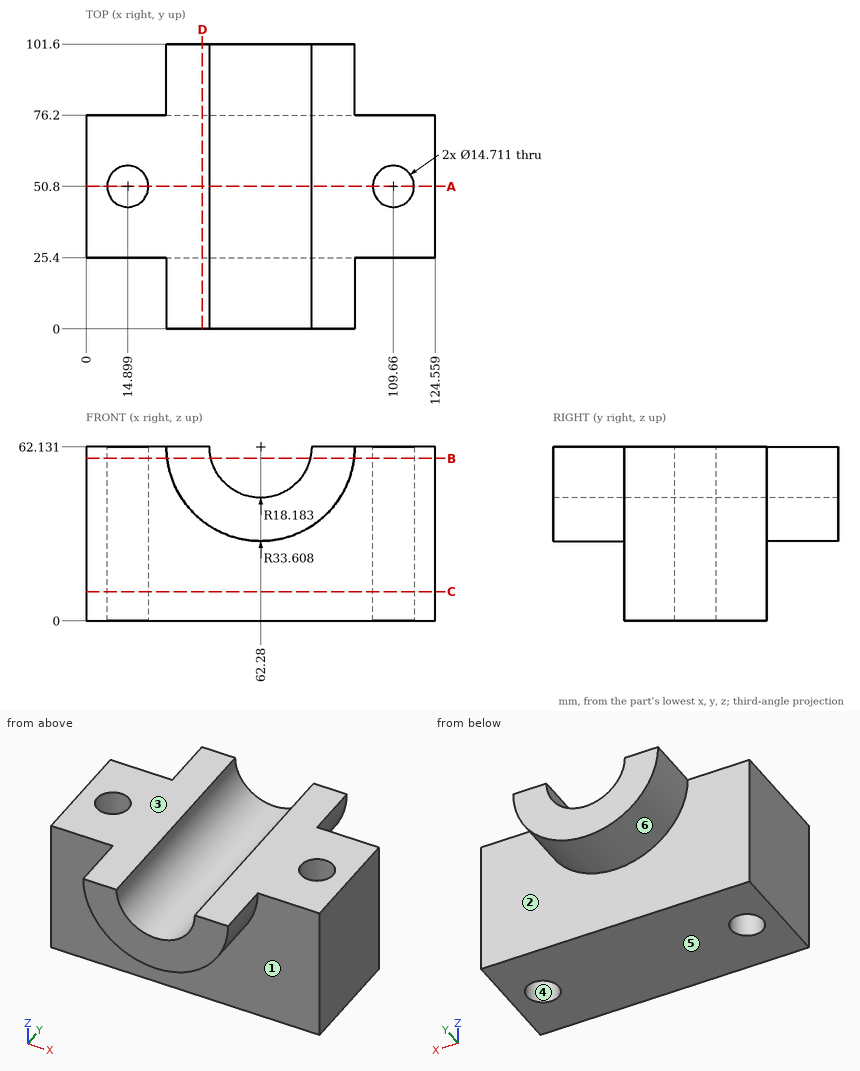
For this review, use the dimensioned drawing (mm, ordinates from the lowest corner) and the shaded views. A direction names the side the tool comes from. Round coordinates to 2 decimals unless told otherwise and drop trailing zeros. Order: outer loops, then holes, each group sorted by start corner. A loop starts at its lowest first (then second) coordinate and runs counter-clockwise, first axis right, second up. Notation, with made-up numbers: (85.25, -26.5) -> (97.25, -26.5) arc R24 ccw to (97.25, -4.5) -> close; hole circle Ø11 at (85, 3). An arc over 180 degrees is marked (long way). Use CSV: the item, a comma, the result in double quotes. Start each with the question number.
(1) Mouldability with a two-part tool opening along X and no side actions: class the marked faces 4, 5 and 6 as pulls with the +X half, pulls with the -X half, needs draft (parallel to the pull), parting line crosses it, or undercut.
(2) Consider section A-A on y = 50.8. Write out the cut boundary in (x, z) (1 decimal).
(3) Consider section D-D on x = 41.5. Write out the cut boundary in (y, z), and give its area (3 significant figures).
(4) Consider section B-B on z = 58. Write out the cut boundary in (x, y) (1 decimal).
(5) Tool access review of the marked faces 1, 2 and 3: name each direction out of +Z, -Z, +X, -X, +Y, -Y from which nothing blocks a thin tool from reaching the whole face with its end or side.
(6) Insertion check: pin 1 (2 mm diameter, centred on x = 71, y = 19, fed in from +Z) (1 decimal); pin 2 (13 mm diameter, centred on x = 109.66, y = 50.8, fed in from +Z); pin 3 (10 mm diameter, centred on y = 19, z = 37.5, fed in from -X); pin 4 (3 mm diameter, centred on x = 17, z = 16, fed in from -Y). Each pin has a flat end and moves straight along its axis. Give the tip position at first contact, or say it passes through.
(7) Wall thickness on probe 1 along X at (y, z) = (50.5, 30.5); probe 2 along X at (y, z) = (57.5, 31) (1 decimal); probe 3 along Y at (x, z) = (16, 40): over which ranges is each line inside the solid? List them lowest first. Write a range as from..to.
(8) Consider section C-C on z = 10.5. Write out the cut boundary in (x, y) (1 decimal).
Responses:
1,face 4,"undercut"
1,face 5,"needs draft"
1,face 6,"parting line crosses it"
2,outline,"(0, 0) -> (7.5, 0) -> (7.5, 62.1) -> (0, 62.1) -> close; (22.3, 0) -> (102.3, 0) -> (102.3, 62.1) -> (80.5, 62.1) arc R18.2 cw to (44.1, 62.1) -> (22.3, 62.1) -> close; (117, 0) -> (124.6, 0) -> (124.6, 62.1) -> (117, 62.1) -> close"
3,outline,"(0, 35.72) -> (25.4, 35.72) -> (25.4, 0) -> (76.2, 0) -> (76.2, 35.72) -> (101.6, 35.72) -> (101.6, 62.13) -> (0, 62.13) -> close"
3,area,"4,500 mm²"
4,outline,"(0, 25.4) -> (28.9, 25.4) -> (28.9, 0) -> (44.6, 0) -> (44.6, 101.6) -> (28.9, 101.6) -> (28.9, 76.2) -> (0, 76.2) -> close; (80, 0) -> (95.6, 0) -> (95.6, 25.4) -> (124.6, 25.4) -> (124.6, 76.2) -> (95.6, 76.2) -> (95.6, 101.6) -> (80, 101.6) -> close; hole circle Ø14.7 at (14.9, 50.8); hole circle Ø14.7 at (109.7, 50.8)"
5,face 1,"-Z, -Y"
5,face 2,"-Z, +Y"
5,face 3,"+Z, +X, -X, +Y, -Y"
6,pin 1,"z = 46.8"
6,pin 2,"through"
6,pin 3,"x = 35"
6,pin 4,"y = 25.4"
7,probe 1,"0..7.55, 22.25..102.31, 117.01..124.56"
7,probe 2,"0..11.9, 17.9..106.6, 112.7..124.6"
7,probe 3,"25.4..43.53, 58.07..76.2"
8,outline,"(0, 25.4) -> (124.6, 25.4) -> (124.6, 76.2) -> (0, 76.2) -> close; hole circle Ø14.7 at (14.9, 50.8); hole circle Ø14.7 at (109.7, 50.8)"
